Autodesk Inventor part; units mm, degrees
ref_plane "YZ Plane" through (0, 0, 0) normal (1, 0, 0) x (0, 1, 0)
ref_plane "XZ Plane" through (0, 0, 0) normal (0, 1, 0) x (-1, 0, 0)
ref_plane "XY Plane" through (0, 0, 0) normal (0, 0, 1) x (1, 0, 0)
sketch "Boceto1" plane through (0, 0, 0) normal (0, 1, 0) x (-1, 0, 0)
  line L0 (28.5, 20.5) -> (-28.5, 20.5)
  line L1 (-28.5, 20.5) -> (-28.5, -20.5)
  line L2 (-28.5, -20.5) -> (28.5, -20.5)
  line L3 (28.5, -20.5) -> (28.5, 20.5)
  line L4 (28.5, 20.5) -> (-28.5, -20.5) construction
  line L5 (-28.5, 20.5) -> (28.5, -20.5) construction
  point P0 (0, 0)
  dimension "d0" = 57
  dimension "d1" = 41
extrude "Extrusión1" add sketch "Boceto1" along normal blind 8
sketch "Boceto2" plane through (0, 8, 0) normal (0, 1, 0) x (1, 0, 0)
  line L0 (28.5, -20.5) -> (28.5, 20.5)
  line L1 (28.5, -20.5) -> (28.5, -17.5)
  line L2 (28.5, -17.5) -> (26.5, -17.5)
  line L3 (26.5, -17.5) -> (26.5, 17.5)
  line L4 (28.5, 20.5) -> (-28.5, 20.5)
  line L5 (26.5, 17.5) -> (-24.5, 17.5)
  line L6 (-24.5, 17.5) -> (-24.5, -17.5)
  line L7 (-24.5, -17.5) -> (26.5, -17.5)
  point P0 (0, 0)
  dimension "d4" = 3
  dimension "d5" = 2
  dimension "d6" = 35
  dimension "d7" = 51
extrude "Extrusión2" cut sketch "Boceto2" against normal blind 6
sketch "Boceto3" plane through (0, 8, 0) normal (0, 1, 0) x (1, 0, 0)
  line L0 (-24.5, -17.5) -> (-24.5, 17.5)
  line L1 (-24.5, -17.5) -> (-28.5, -17.5)
  line L2 (-28.5, 20.5) -> (-28.5, -20.5)
  line L3 (-28.5, -17.5) -> (-28.5, 17.5)
  line L4 (-24.5, 17.5) -> (26.5, 17.5)
  line L5 (-28.5, 17.5) -> (-24.5, 17.5)
  line L6 (-24.5, 17.5) -> (-24.5, -17.5)
  point P0 (0, 0)
  dimension "d10" = 35
extrude "Extrusión3" cut sketch "Boceto3" against normal blind 6
sketch "Boceto4" plane through (-28.5, 0, -20.5) normal (-1, 0, 0) x (0, 0, 1)
  line L0 (3, 8) -> (38, 8)
  line L1 (3, 8) -> (3, 7)
  line L2 (3, 7) -> (2, 7)
  line L3 (2, 7) -> (2, 6)
  line L4 (2, 6) -> (3, 6)
  line L5 (3, 8) -> (3, 2)
  line L6 (3, 6) -> (3, 7)
  point P0 (20.5, 0)
  dimension "d13" = 1
  dimension "d14" = 1
  dimension "d15" = 1
extrude "Extrusión4" cut sketch "Boceto4" against normal blind 55
sketch "Boceto5" plane through (-28.5, 0, -20.5) normal (-1, 0, 0) x (0, 0, 1)
  line L0 (3, 8) -> (38, 8)
  line L1 (38, 8) -> (38, 7)
  line L2 (38, 8) -> (38, 2)
  line L3 (38, 7) -> (39, 7)
  line L4 (39, 7) -> (39, 6)
  line L5 (39, 6) -> (38, 6)
  line L6 (38, 7) -> (38, 6)
  point P0 (20.5, 0)
  dimension "d18" = 1
  dimension "d19" = 1
  dimension "d20" = 1
extrude "Extrusión5" cut sketch "Boceto5" against normal blind 55
sketch "Boceto6" plane through (-28.5, 0, -20.5) normal (-1, 0, 0) x (0, 0, 1)
  line L0 (3, 8) -> (3, 7)
  line L1 (3, 8) -> (3, 6)
  line L2 (3, 6) -> (1, 6)
  line L3 (1, 6) -> (1, 7)
  line L4 (2, 6) -> (2, 7)
  line L5 (1, 7) -> (2, 7)
  line L6 (2, 7) -> (2, 8)
  line L7 (0, 8) -> (3, 8)
  line L8 (3, 8) -> (2, 8)
  point P0 (20.5, 0)
  dimension "d23" = 2
  dimension "d24" = 2
  dimension "d25" = 1
extrude "Extrusión6" cut sketch "Boceto6" against normal blind 55
sketch "Boceto7" plane through (-28.5, 0, -20.5) normal (-1, 0, 0) x (0, 0, 1)
  line L0 (2, 8) -> (38, 8)
  line L1 (39, 6) -> (38, 6)
  line L2 (38, 8) -> (38, 6)
  line L3 (38, 6) -> (40, 6)
  line L4 (40, 6) -> (40, 7)
  line L5 (38, 7) -> (39, 7)
  line L6 (40, 7) -> (39, 7)
  line L7 (39, 7) -> (39, 8)
  line L8 (38, 8) -> (41, 8)
  line L9 (38, 8) -> (39, 8)
  point P0 (20.5, 0)
  dimension "d28" = 2
  dimension "d29" = 1
extrude "Extrusión7" cut sketch "Boceto7" against normal blind 55
sketch "Boceto8" plane through (26.5, 2, -17.5) normal (-1, 0, 0) x (0, 0, 1)
  line L0 (-1, 6) -> (36, 6)
  line L1 (-1, 5) -> (-1, 6)
  line L2 (-1, 6) -> (-1, 5)
  line L3 (-2, 4) -> (-2, 5)
  line L4 (-1, 5) -> (-2, 5)
  line L5 (-2, 5) -> (-2, 4)
  line L6 (0, 4) -> (-2, 4)
  line L7 (-2, 4) -> (0, 4)
  line L8 (0, 0) -> (0, 4)
  line L9 (0, 4) -> (0, 0)
  line L10 (35, 4) -> (35, 0)
  line L11 (0, 0) -> (35, 0)
  line L12 (35, 0) -> (35, 4)
  line L13 (37, 4) -> (35, 4)
  line L14 (35, 4) -> (37, 4)
  line L15 (37, 5) -> (37, 4)
  line L16 (37, 4) -> (37, 5)
  line L17 (36, 5) -> (37, 5)
  line L18 (37, 5) -> (36, 5)
  line L19 (36, 6) -> (36, 5)
  line L20 (36, 5) -> (36, 6)
  line L21 (36, 6) -> (-1, 6)
  point P0 (17.5, -2)
extrude "Extrusión8" cut sketch "Boceto8" against normal blind 1
sketch "Boceto9" plane through (-28.5, 0, -20.5) normal (-1, 0, 0) x (0, 0, 1)
  line L0 (3, 2) -> (3, 6)
  line L1 (3, 6) -> (3, 2)
  line L2 (38, 2) -> (3, 2)
  line L3 (3, 2) -> (38, 2)
  line L4 (38, 6) -> (38, 2)
  line L5 (38, 2) -> (38, 6)
  line L6 (38, 6) -> (3, 6)
  point P0 (20.5, 0)
extrude "Extrusión9" add sketch "Boceto9" against normal blind 4
sketch "Boceto10" plane through (-28.5, 0, -20.5) normal (-1, 0, 0) x (0, 0, 1)
  line L0 (0, 0) -> (41, 0)
  line L1 (0, 0) -> (42, 0)
  line L2 (42, 0) -> (42, 8)
  line L3 (42, 8) -> (42, 9)
  line L4 (42, 9) -> (40, 9)
  line L5 (40, 9) -> (40, 7)
  line L6 (40, 7) -> (41, 7)
  line L7 (41, 0) -> (41, 8)
  line L8 (41, 7) -> (41, 5)
  line L9 (41, 5) -> (0, 5)
  line L10 (0, 0) -> (0, 8)
  line L11 (0, 5) -> (0, 7)
  line L12 (1, 7) -> (2, 7)
  line L13 (0, 7) -> (1, 7)
  line L14 (1, 7) -> (1, 9)
  line L15 (1, 9) -> (-1, 9)
  line L16 (-1, 9) -> (-1, 0)
  line L17 (-1, 0) -> (0, 0)
  point P0 (20.5, 0)
  dimension "d36" = 42
  dimension "d37" = 8
  dimension "d38" = 1
  dimension "d39" = 2
  dimension "d40" = 2
  dimension "d41" = 2
extrude "Extrusión10" add sketch "Boceto10" against normal blind 57
sketch "Boceto11" plane through (-28.5, 6, -19.5) normal (-1, 0, 0) x (0, 0, 1)
  line L0 (39, 2) -> (0, 2)
  line L1 (39, 2) -> (39, 1)
  line L2 (38, 1) -> (39, 1)
  line L3 (39, 1) -> (38, 1)
  line L4 (38, 2) -> (38, 1)
  line L5 (38, 1) -> (38, 2)
  line L6 (38, 2) -> (39, 2)
  line L7 (0, 1) -> (1, 1)
  line L8 (0, 1) -> (0, 2)
  line L9 (1, 1) -> (1, 2)
  line L10 (0, 2) -> (1, 2)
  line L11 (1, 2) -> (1, 1)
  line L12 (0, 0) -> (0, 1)
  line L13 (1, 1) -> (0, 1)
  line L14 (0, 1) -> (-1, 1)
  line L15 (-1, 1) -> (-1, -1)
  line L16 (-1, -1) -> (40, -1)
  line L17 (41, 3) -> (41, -6)
  line L18 (40, -1) -> (40, 1)
  line L19 (40, 1) -> (39, 1)
  line L20 (0, 1) -> (1, 1)
  line L21 (0, 0) -> (0, 1)
  line L22 (0, 1) -> (0, 0)
  line L23 (0, 0) -> (39, 0)
  line L24 (39, 0) -> (39, 1)
  line L25 (39, 1) -> (39, 0)
  line L26 (39, 1) -> (39, 0)
  point P0 (19.5, -6)
  dimension "d44" = 1
  dimension "d45" = 2
  dimension "d46" = 41
extrude "Extrusión11" cut sketch "Boceto11" against normal blind 56 contours L1 L2 L4 L0 | L19 L18 L16 L15 L14 L12 L23 L24 | L9 L7 L8 L0
sketch "Boceto12" plane through (28.5, 0, 21.5) normal (1, 0, 0) x (0, 0, -1)
  line L0 (2, 8) -> (2, 9)
  line L1 (41, 9) -> (41, 8)
  line L2 (2, 8) -> (41, 8)
  line L3 (41, 8) -> (41, 9)
  line L4 (41, 9) -> (2, 9)
  line L5 (2, 9) -> (2, 8)
  point P0 (21.5, 0)
extrude "Extrusión12" add sketch "Boceto12" against normal blind 1
sketch "Boceto13" plane through (-28.5, 5, 20.5) normal (0, 1, 0) x (1, 0, 0)
  line L0 (56, 1) -> (56, 0)
  line L1 (0, 40) -> (56, 40)
  line L2 (56, 1) -> (4, 1)
  line L3 (4, 1) -> (4, 40)
  line L4 (4, 40) -> (56, 40)
  line L5 (56, 40) -> (56, 1)
  point P0 (28.5, 20.5)
  dimension "d51" = 52
extrude "Extrusión13" cut sketch "Boceto13" against normal blind 4
sketch "Boceto14" plane through (-28.5, 0, -21.5) normal (-1, 0, 0) x (0, 0, 1)
  line L0 (41, 9) -> (2, 9)
  line L1 (41, 9) -> (40.25, 9)
  line L2 (40.25, 9) -> (40.25, 7)
  line L3 (40.25, 7) -> (41.5, 7)
  line L4 (41, 7) -> (42, 7)
  line L5 (41.5, 7) -> (41.5, 5)
  line L6 (41, 5) -> (42, 5)
  line L7 (41.5, 5) -> (1.5, 5)
  line L8 (41, 5) -> (2, 5)
  line L9 (1.5, 5) -> (1.5, 7)
  line L10 (1, 7) -> (2, 7)
  line L11 (1.5, 7) -> (2.75, 7)
  line L12 (2.75, 7) -> (2.75, 9)
  line L13 (0, 9) -> (43, 9)
  line L14 (2.75, 9) -> (0, 9)
  line L15 (0, 0) -> (0, 9)
  line L16 (0, 9) -> (0, 0)
  line L17 (43, 9) -> (43, 0)
  line L18 (0, 0) -> (43, 0)
  line L19 (43, 0) -> (43, 9)
  line L20 (43, 9) -> (40.25, 9)
  point P0 (21.5, 0)
  point P1 (2, 7)
  dimension "d54" = 0.75
  dimension "d55" = 2
  dimension "d56" = 40
  dimension "d57" = 1.25
extrude "Extrusión14" add sketch "Boceto14" against normal blind 4 contours L13 L17 L18 L15 L0 L12 L11 L10 L9 L7 L6 L5 L3 L2
sketch "Boceto15" plane through (-24.5, 0, -21.5) normal (1, 0, 0) x (0, 0, -1)
  line L0 (-2.75, 9) -> (-2.75, 7)
  line L1 (-2.75, 9) -> (-2, 9)
  line L2 (-2, 9) -> (-2, 7)
  line L3 (-2.75, 7) -> (-2, 7)
  line L4 (-2, 7) -> (-2.75, 7)
  line L5 (-2.75, 7) -> (-2.75, 9)
  line L6 (-1, 5) -> (-1.5, 5)
  line L7 (-1.5, 5) -> (-1, 5)
  line L8 (-1, 7) -> (-1, 5)
  line L9 (-1, 5) -> (-1, 7)
  line L10 (-1, 7) -> (-1.5, 7)
  line L11 (-1.5, 7) -> (-1.5, 5)
  line L12 (-1.5, 7) -> (-1.5, 5)
  line L13 (-41, 7) -> (-41, 9)
  line L14 (-40.25, 9) -> (-41, 9)
  line L15 (-41, 9) -> (-40.25, 9)
  line L16 (-40.25, 7) -> (-40.25, 9)
  line L17 (-40.25, 9) -> (-40.25, 7)
  line L18 (-41, 7) -> (-40.25, 7)
  line L19 (-40.25, 7) -> (-41, 7)
  line L20 (-41, 7) -> (-41, 9)
  line L21 (-41.5, 5) -> (-42, 5)
  line L22 (-41.5483, 5) -> (-42, 5)
  line L23 (-42, 5) -> (-42, 7)
  line L24 (-42, 5) -> (-42, 7)
  line L25 (-42, 7) -> (-41.5, 7)
  line L26 (-42, 7) -> (-41.5, 7)
  line L27 (-41.5, 5) -> (-41.5, 7)
  line L28 (-41.5, 7) -> (-41.5, 5)
  point P0 (-21.5, 0)
extrude "Extrusión15" add sketch "Boceto15" along normal blind 53
properties part number "TapaCajaArduinoNano"
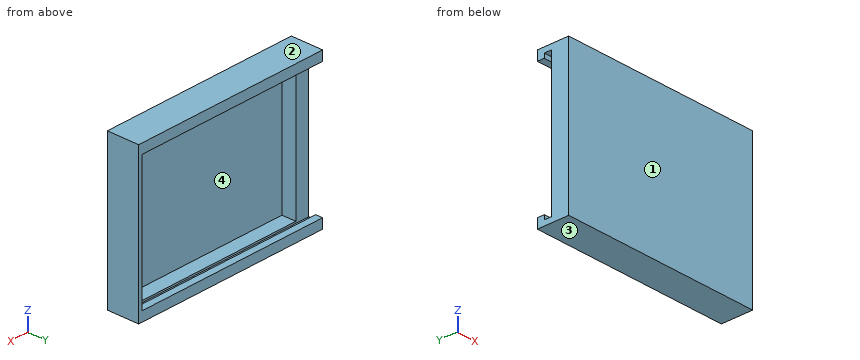
Work out the finished part from the listing and answer in its coordinate system (mm). Face numbers are marked on the shaded views. Round coordinates to 2 decimals unless told otherwise and drop trailing zeros. Loops run counter-clockwise (first coordinate to the right, second up) from the corner with the lowest first, then second, coordinate; pieces in that order, holes last. Notation, with made-up numbers: (42.25, -19.5) - (73.25, -19.5) arc R19 ccw to (73.25, -10.5) - close; hole circle Ø3 at (50, 70.25). An arc over 180 degrees is marked (long way). Use one line per item in the form item = value. Start each with the question number.
(1) A flat-ended cylindrical pin translates along its axis: P1, Ø8, axis at x = 5.5, z = 11, coming from the +Y side. Find the tip coordinate at first contact, or state that the pin passes through.
(2) Consider line 1 (Z direction, x = 24, y = 2); line 2 (Z direction, x = -18, y = 5.25); line 3 (X direction, y = 4.75, z = -2.5). Determine where each line is inside the solid, lowest interval first.
(3) Find section B-B on y = 1.75. Determine the outline of the cut face in (x, z), and give its area (3 significant figures).
(4) Find section D-D on x = -15. Determine the outline of the cut face in (y, z).
(5) Find section C-C on y = 8. Determine the outline of the cut face in (x, z).
(6) Determine the mould class of the marked faces 1, 2, 3 and 4 for opening direction Z: +Z half, -Z half, draft (parallel to the pull), parting line (faces both ways), or undercut.
(7) Find section A-A on z = -12. Determine the outline of the cut face in (x, y).
Answer list:
q1.P1 = 1
q2.line_1 = -21.5 to -19.5, 19.5 to 21.5
q2.line_2 = -21.5 to -20, 20 to 21.5
q2.line_3 = -28.5 to -24.5, 27.5 to 28.5
q3.outline = (-28.5, -21.5) - (28.5, -21.5) - (28.5, 21.5) - (-28.5, 21.5) - close; hole (-24.5, -19.5) - (27.5, -19.5) - (27.5, 19.5) - (-24.5, 19.5) - close
q3.area = 423 mm^2
q4.outline = (0, -21.5) - (9, -21.5) - (9, -18.75) - (7, -18.75) - (7, -20) - (5, -20) - (5, -19.5) - (1, -19.5) - (1, 19.5) - (5, 19.5) - (5, 20) - (7, 20) - (7, 18.75) - (9, 18.75) - (9, 21.5) - (0, 21.5) - close
q5.outline = (-28.5, -21.5) - (28.5, -21.5) - (28.5, 21.5) - (-28.5, 21.5) - (-28.5, 18.75) - (27.5, 18.75) - (27.5, -18.75) - (-28.5, -18.75) - close
q6.face_1 = draft
q6.face_2 = +Z half
q6.face_3 = -Z half
q6.face_4 = undercut
q7.outline = (-28.5, 0) - (28.5, 0) - (28.5, 9) - (27.5, 9) - (27.5, 1) - (-24.5, 1) - (-24.5, 5) - (-28.5, 5) - close
